The model under review builds one solid part; all positions refer to its coordinate system, in mm. Coordinates: 2 decimals unless noted, no trailing zeros. Loops run counter-clockwise (first coordinate to the right, second up) from the corner with the lowest first, then second, coordinate; pieces in that order, holes last. Notation, with made-up numbers: (67.5, 76.5) - (103.5, 76.5) arc R25 ccw to (103.5, 88.5) - close; hole circle Ø7 at (-38, -35.5). An arc over 180 degrees is marked (long way). Answer in a Markdown table with one row per item. Add a question column.
(1) We need section B-B on y = 12. Write out the cut boundary in (x, z).
(2) We need section D-D on z = 0. Write out the cut boundary in (x, y).
(3) Mouldability with a two-part tool opening along Y and no side actions: class faces 1 (the cylindrical face through (12.19, 12.45, -1.43)), 2 (the cylindrical face through (0.2, 1.33, 6.51)), 3 (the flat face through (14, 12, 2)) as +Y half, -Y half, draft (parallel to the pull), parting line (faces both ways), or undercut.
(4) For line 1 along Y through (x, z) = (9, 2.75); line 2 along Y through (x, z) = (12.1, 0); line 3 along Z through (x, y) = (11.1, 12), list the stretches that pass through material, from the lowest coordinate up.
(5) We need section A-A on x = 9. Write out the cut boundary in (y, z).
(6) For P1, Ø1.8, axis at y = 12, z = 0, coming from the +X side; P2, Ø1, axis at x = -0.5, z = -6, coming from the +Y side (3 decimals); P3, Ø6, axis at x = 10.5, z = -7, coming from the +Y side, all flat-tipped, find the tip position at first contact; note any pin that passes through.
(7) We need section C-C on z = 3. Write out the cut boundary in (x, y).
Autodesk Inventor part; units mm, degrees
ref_plane "YZ Plane" through (0, 0, 0) normal (1, 0, 0) x (0, 1, 0)
ref_plane "XZ Plane" through (0, 0, 0) normal (0, 1, 0) x (-1, 0, 0)
ref_plane "XY Plane" through (0, 0, 0) normal (0, 0, 1) x (1, 0, 0)
sketch "Sketch1" plane through (0, 0, 0) normal (0, 1, 0) x (-1, 0, 0)
  line L0 (14, 9) -> (-14, 9)
  line L1 (-14, 9) -> (-14, -9)
  line L2 (-14, -9) -> (14, -9)
  line L3 (14, -9) -> (14, 9)
  line L4 (0, 0) -> (0, -9) construction
  line L5 (0, 0) -> (-14, 0) construction
  dimension "d0" = 18
  dimension "d1" = 28
extrude "Extrusion1" add sketch "Sketch1" along normal blind 24
sketch "Sketch4" plane through (-14, 0, 9) normal (0, 0, 1) x (1, 0, 0)
  line L0 (0, 0) -> (0, 24) construction
  line L1 (0, 12) -> (31.0841, 12) construction
  circle A0 centre (23, 12) radius 2
  line L2 (28, 0) -> (28, 24)
  point P0 (14, 0)
  dimension "d4" = 4
  dimension "d5" = 5
extrude "Extrusion2" cut sketch "Sketch4" against normal up to next
sketch "Sketch5" plane through (14, 0, 9) normal (1, 0, 0) x (0, 0, -1)
  circle A0 centre (9, 12) radius 1.5
  line L0 (0, 0) -> (0, 24) construction
  line L1 (0, 12) -> (9.7328, 12) construction
  line L2 (9, 0) -> (9, 12) construction
  circle A1 centre (9, 12) radius 12.5
  circle A2 centre (9, 12) radius 15
  dimension "d8" = 3
  dimension "d9" = 25
  dimension "d10" = 30
extrude "Extrusion3" cut sketch "Sketch5" against normal up to next
sketch "Sketch6" plane through (0, 24, 0) normal (0, 1, 0) x (1, 0, 0)
  line L0 (0, 0) -> (30, 0) construction
  dimension "d13" = 30
properties part number "motor_quick"
Outcome:
| question | item | result |
|---|---|---|
| 1 | outline | (-14, -9) - (7, -9) - (7, 9) - (-14, 9) - close; (11, -9) - (14, -9) - (14, -1.5) - (11, -1.5) - close; (11, 1.5) - (14, 1.5) - (14, 9) - (11, 9) - close |
| 2 | outline | (-14, 0) - (14, 0) - (14, 10.5) - (10.32, 10.5) arc R2 cw (long way) to (10.32, 13.5) - (14, 13.5) - (14, 24) - (-14, 24) - close |
| 3 | face 1 | undercut |
| 3 | face 2 | -Y half |
| 3 | face 3 | draft |
| 4 | line 1 | 0 to 10, 14 to 24 |
| 4 | line 2 | 0 to 10.5, 13.5 to 24 |
| 4 | line 3 | -9 to -1.5, 1.5 to 9 |
| 5 | outline | (0, -3.5) arc R12.5 ccw to (3.33, -9) - (10, -9) - (10, 9) - (3.33, 9) arc R12.5 ccw to (0, 3.5) - close; (14, -9) - (20.67, -9) arc R12.5 ccw to (24, -3.5) - (24, 3.5) arc R12.5 ccw to (20.67, 9) - (14, 9) - close |
| 6 | P1 | x = 7.21 |
| 6 | P2 | y = 23.225 |
| 6 | P3 | y = 23.84 |
| 7 | outline | (-14, 0) - (14, 0) - (14, 24) - (-14, 24) - close; hole circle Ø4 at (9, 12) |
